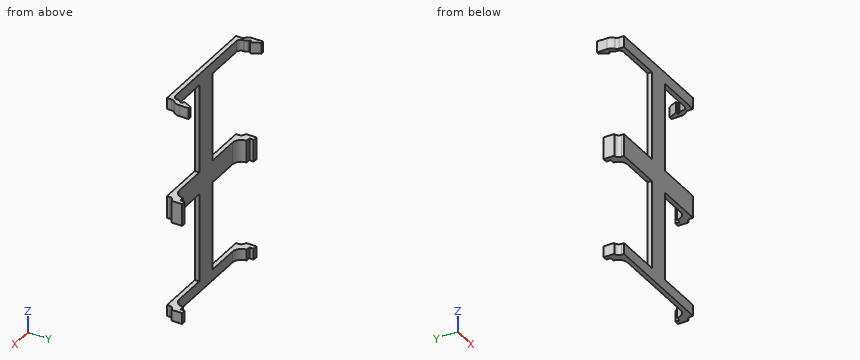
```python
from build123d import *

# Parameters (mm, degrees)
BOSS_EXTRUDE1_DEPTH = 63.5
CUT_EXTRUDE1_REACH  = 72.818
SKETCH2_W           = 14.605
SKETCH2_H           = 25.4
BOSS_EXTRUDE2_DEPTH = 3.175
CUT_EXTRUDE2_REACH  = 72.98
SKETCH4_W           = 0.588974589
SKETCH4_H           = 2.54
FILLET1_R           = 2.38
FILLET2_R           = 1.27
FILLET3_R           = 2.54
FILLET5_R           = 1.27
FILLET6_R           = 1.27


# Some blends are built 0.0001 mm under size
with BuildPart() as part:
    # Sketch1 → Boss-Extrude1 (new body)
    with BuildSketch(Plane.XY):
        Polygon((0, 0), (13.158113026, 0), (13.158113026, 1.27), (-2.081886974, 1.27), (-2.081886974, 3.81), (-3.351886974, 3.81), (-3.351886974, 5.08), (-4.621886974, 5.08), (-4.621886974, 2.032), (-3.351886974, 2.032), (-3.351886974, 0), align=None)
    boss_extrude1 = extrude(amount=-BOSS_EXTRUDE1_DEPTH)

    # Mirror1: Boss-Extrude1 across plane
    add(boss_extrude1.mirror(Plane(origin=(13.158113026, 1.27, -63.5), x_dir=(0, 0, 1), z_dir=(-1, 0, 0))))

    # Cut-Extrude1: up to this face of the body (flat: up to its plane)
    cut_extrude1_end = Plane(part.part.faces().sort_by_distance((13.158113026, 0, -31.75))[0])
    # Sketch2 → Cut-Extrude1 (cut, up to the picked face)
    with BuildSketch(Plane(origin=(0, 5.08, 0), x_dir=(1, 0, 0), z_dir=(0, 1, 0)), mode=Mode.PRIVATE) as cut_extrude1_sk1:
        with Locations((2.680613026, 15.875)):
            Rectangle(SKETCH2_W, SKETCH2_H)
    cut_extrude1_tool1 = split(extrude(cut_extrude1_sk1.sketch, amount=-CUT_EXTRUDE1_REACH, mode=Mode.PRIVATE), bisect_by=cut_extrude1_end, keep=Keep.BOTH, mode=Mode.PRIVATE)
    # Sketch2 → Cut-Extrude1 (cut, up to the picked face)
    with BuildSketch(Plane(origin=(0, 5.08, 0), x_dir=(1, 0, 0), z_dir=(0, 1, 0)), mode=Mode.PRIVATE) as cut_extrude1_sk2:
        with Locations((23.635613026, 15.875)):
            Rectangle(SKETCH2_W, SKETCH2_H)
    cut_extrude1_tool2 = split(extrude(cut_extrude1_sk2.sketch, amount=-CUT_EXTRUDE1_REACH, mode=Mode.PRIVATE), bisect_by=cut_extrude1_end, keep=Keep.BOTH, mode=Mode.PRIVATE)
    # Sketch2 → Cut-Extrude1 (cut, up to the picked face)
    with BuildSketch(Plane(origin=(0, 5.08, 0), x_dir=(1, 0, 0), z_dir=(0, 1, 0)), mode=Mode.PRIVATE) as cut_extrude1_sk3:
        with Locations((2.680613026, 47.625)):
            Rectangle(SKETCH2_W, SKETCH2_H)
    cut_extrude1_tool3 = split(extrude(cut_extrude1_sk3.sketch, amount=-CUT_EXTRUDE1_REACH, mode=Mode.PRIVATE), bisect_by=cut_extrude1_end, keep=Keep.BOTH, mode=Mode.PRIVATE)
    # Sketch2 → Cut-Extrude1 (cut, up to the picked face)
    with BuildSketch(Plane(origin=(0, 5.08, 0), x_dir=(1, 0, 0), z_dir=(0, 1, 0)), mode=Mode.PRIVATE) as cut_extrude1_sk4:
        with Locations((23.635613026, 47.625)):
            Rectangle(SKETCH2_W, SKETCH2_H)
    cut_extrude1_tool4 = split(extrude(cut_extrude1_sk4.sketch, amount=-CUT_EXTRUDE1_REACH, mode=Mode.PRIVATE), bisect_by=cut_extrude1_end, keep=Keep.BOTH, mode=Mode.PRIVATE)
    add(cut_extrude1_tool1.solids().sort_by(Axis((2.680613, 5.08, -15.875), (0, -1, 0)))[0], mode=Mode.SUBTRACT)
    add(cut_extrude1_tool2.solids().sort_by(Axis((23.635613, 5.08, -15.875), (0, -1, 0)))[0], mode=Mode.SUBTRACT)
    add(cut_extrude1_tool3.solids().sort_by(Axis((2.680613, 5.08, -47.625), (0, -1, 0)))[0], mode=Mode.SUBTRACT)
    add(cut_extrude1_tool4.solids().sort_by(Axis((23.635613, 5.08, -47.625), (0, -1, 0)))[0], mode=Mode.SUBTRACT)

    # Sketch3 → Boss-Extrude2 (add)
    with BuildSketch(Plane.XY):
        Polygon((-4.621886974, 4.445), (-2.637712851, 4.445), (-3.870360235, 6.985), (-4.621886974, 6.985), align=None)
    boss_extrude2 = extrude(amount=-BOSS_EXTRUDE2_DEPTH)

    # Mirror2: Boss-Extrude2 across plane
    add(boss_extrude2.mirror(Plane.ZY.offset(-13.158113026)))

    # Sketch4 → Cut-Extrude2 (cut, up to next)
    with BuildSketch(Plane.XY, mode=Mode.PRIVATE) as cut_extrude2_sk1:
        with Locations((-2.376374269, 2.54)):
            Rectangle(SKETCH4_W, SKETCH4_H)
    cut_extrude2_tool1 = extrude(cut_extrude2_sk1.sketch, amount=-CUT_EXTRUDE2_REACH, mode=Mode.PRIVATE) & part.part
    cut_extrude2 = cut_extrude2_tool1.solids().sort_by_distance((-2.376374, 2.54, 0))[0]
    add(cut_extrude2, mode=Mode.SUBTRACT)

    # Mirror3: Cut-Extrude2 across plane
    add(cut_extrude2.mirror(Plane.ZY.offset(-13.158113026)), mode=Mode.SUBTRACT)

    # Fillet1
    # the kernel refuses this fillet: 2.38 mm, written as the material it takes off along each edge
    with BuildSketch(Plane(origin=(30.938113026, 2.032, 5.263257071), x_dir=(0, 1, 0), z_dir=(0, 0, -1))) as fillet1_piece_1:
        with BuildLine():
            CenterArc((2.105302829, -2.38), FILLET1_R, 90, 62.200005552)
            Line((0, -1.27), (-0.042106057, -1.2478))
            ThreePointArc((-0.042106057, -1.2478), (-0.0476, -0.635), (-0.0476, 0))
            Line((-0.0476, 0), (0, 0.0476))
            Line((0, 0.0476), (2.105302829, 0.0476))
            Line((2.105302829, 0.0476), (2.105302829, 0))
        make_face()
    extrude(amount=13.701514143, mode=Mode.SUBTRACT)
    with BuildSketch(Plane(origin=(-4.621886974, 2.032, 5.263257071), x_dir=(1, 0, 0), z_dir=(0, 0, -1))) as fillet1_piece_2:
        with BuildLine():
            CenterArc((2.38, -2.105302829), FILLET1_R, 117.799994448, 62.200005552)
            Line((0, -2.105302829), (-0.0476, -2.105302829))
            Line((-0.0476, -2.105302829), (-0.0476, 0))
            Line((-0.0476, 0), (0, 0.0476))
            ThreePointArc((0, 0.0476), (0.635, 0.0476), (1.2478, 0.042106057))
            Line((1.2478, 0.042106057), (1.27, 0))
        make_face()
    extrude(amount=13.701514143, mode=Mode.SUBTRACT)

    # Fillet2
    # the kernel refuses this fillet: 1.27 mm, written as the material it adds along each edge
    with BuildSketch(Plane(origin=(-3.351886974, 2.032, 0), x_dir=(0, -1, 0), z_dir=(0, 0, -1))) as fillet2_piece_1:
        with BuildLine():
            CenterArc((0.662024402, 1.27), FILLET2_R, 220.696704321, 49.303295679)
            ThreePointArc((-0.30085384, 0.441890411), (-0.137980638, 0.229419053), (0, 0))
            Line((0, 0), (0.662024402, 0))
        make_face()
    extrude(amount=3.175)
    with BuildSketch(Plane(origin=(29.668113026, 2.032, 0), x_dir=(0, -1, 0), z_dir=(0, 0, -1))) as fillet2_piece_2:
        with BuildLine():
            CenterArc((0.662024402, -1.27), FILLET2_R, 90, 49.303295679)
            ThreePointArc((-0.30085384, -0.441890411), (-0.137980638, -0.229419053), (0, 0))
            Line((0, 0), (0.662024402, 0))
        make_face()
    extrude(amount=3.175)
    # the kernel refuses this fillet: 1.27 mm, written as the material it takes off along each edge
    with BuildSketch(Plane(origin=(28.987087615, 3.81, 2.81292656), x_dir=(0, -1, 0), z_dir=(0, 0, -1))) as fillet2_2_piece_1:
        with BuildLine():
            CenterArc((1.125170624, -1.27), FILLET2_R, 90, 62.370030247)
            Line((0, -0.681025411), (0, 0))
            Line((0, 0), (1.125170624, 0))
        make_face()
    extrude(amount=8.800853121, mode=Mode.SUBTRACT)
    with BuildSketch(Plane(origin=(-2.670861563, 3.81, 2.81292656), x_dir=(-1, 0, 0), z_dir=(0, 0, -1))) as fillet2_2_piece_2:
        with BuildLine():
            CenterArc((1.27, -1.125170624), FILLET2_R, 117.629969753, 62.370030247)
            Line((0, -1.125170624), (0, 0))
            Line((0, 0), (0.681025411, 0))
        make_face()
    extrude(amount=8.800853121, mode=Mode.SUBTRACT)

    # Fillet3
    fillet3_edges = [part.edges().sort_by_distance(p)[0] for p in [
        (28.398113026, 1.27, -31.75),
        (28.398113026, 1.27, -61.9125),
        (-2.081886974, 1.27, -61.9125),
        (-2.081886974, 1.27, -31.75),
    ]]
    fillet(fillet3_edges, radius=FILLET3_R - 0.0001)  # a hair under: the kernel refuses the full size

    # Fillet5
    fillet5_edges = [part.edges().sort_by_distance(p)[0] for p in [
        (29.668113026, 2.032, -61.9125),
        (29.668113026, 2.032, -31.75),
        (-3.351886974, 2.032, -61.9125),
        (-3.351886974, 2.032, -31.75),
    ]]
    fillet(fillet5_edges, radius=FILLET5_R - 0.0001)  # a hair under: the kernel refuses the full size

    # Fillet6
    fillet6_edges = [part.edges().sort_by_distance(p)[0] for p in [
        (-2.670861563, 1.27, -1.5875),
        (28.987087615, 1.27, -1.5875),
    ]]
    fillet(fillet6_edges, radius=FILLET6_R)


solid = part.part
```
CAD build for the part. Positions are in the model's coordinates, mm. Give positions to 0.01 mm unless a question says otherwise; leave off trailing zeros. Loops run counter-clockwise (first coordinate to the right, second up) from the corner with the lowest first, then second, coordinate; pieces in that order, holes last. Notation, with made-up numbers: M 30,-19.75 L 72,-19.75 A26 ccw 72,4.25 Z; hole C -34,69 d1. An arc over 180 degrees is marked long. Use one line per item in the form item = value.
Item 1: Slice it at A-A (x = 22). List the corners of the cut face in (y, z) (3 decimals).
Determined:
outline = M 0,-63.5 L 1.27,-63.5 L 1.27,-60.325 L 0,-60.325 Z; M 0,-34.925 L 1.27,-34.925 L 1.27,-28.575 L 0,-28.575 Z; M 0,-3.175 L 1.27,-3.175 L 1.27,0 L 0,0 Z
Item 2: Drill centre lines: probe 1 along Z at (x, y) = (16.5, 0.75) (3 decimals); probe 2 along X at (y, z) = (1, -44.5); probe 3 along X at (y, z) = (2.25, -30). Where is each one in solid material? Low to high. Write a range as from..to.
Determined:
probe_1 = -63.5..-60.325, -34.925..-28.575, -3.175..0
probe_2 = 9.98..16.33
probe_3 = -4.62..-1.55, 27.86..30.94
Item 3: Flat gauge pins, fed straight in: pin 1 (0.6 mm diameter, centred on y = 0.5, z = -30.5, fed in from +X); pin 2 (4 mm diameter, centred on y = 2, z = -54, fed in from -X); pin 3 (1 mm diameter, centred on x = 29, z = -31, fed in from +Y); pin 4 (1 mm diameter, centred on x = -0.5, y = 4, fed in from +Z). Where does each tip first touch, or does it go through?
Determined:
pin_1 = 29.67
pin_2 = 9.98
pin_3 = 3.81
pin_4 = through
Item 4: Slice it at C-C (z = -10.5). List the corners of the cut face in (x, y), plus the area to 3 significant figures.
Determined:
outline = M 9.98,0 L 16.33,0 L 16.33,1.27 L 9.98,1.27 Z
area = 8.06 mm2
